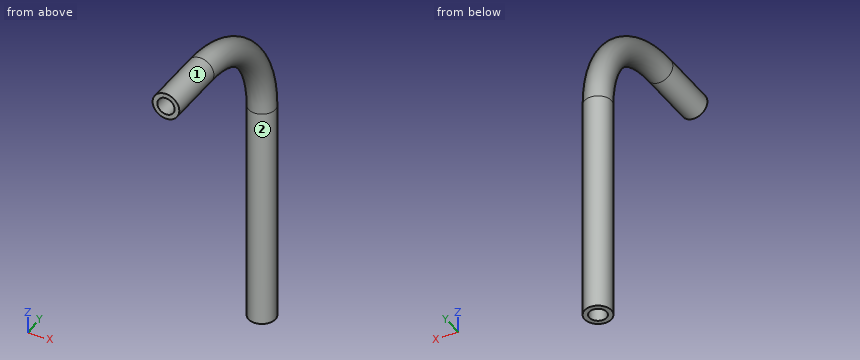
from build123d import *

# Parameters (mm, degrees)
F0_R   = 2
F0_R_2 = 1.3


with BuildPart() as f2:
    # F2: sweep along a path in F1
    with BuildLine(Plane.YZ) as f2_path:
        Line((0, 0), (0, 34))
        ThreePointArc((0, 34), (-4.686291501, 45.313708499), (-16, 50))
        Line((-16, 50), (-25, 50))
    # F0 (on Top) → F2 (sweep)
    with BuildSketch(Plane.XY):
        Circle(F0_R)
        Circle(F0_R_2, mode=Mode.SUBTRACT)
    sweep(path=f2_path.line)


solid = f2.part
Verification items for the finished model (mm, model axes). Face numbers are marked on the shaded views. A direction names the side the tool comes from. Give positions to 0.01 mm unless a question says otherwise; leave off trailing zeros. Write each loop counter-clockwise with the first axis right and the second up, starting at its lowest first coordinate (ties: lowest second). Pieces come first, ordered by that corner, then holes. Notation, with made-up numbers: M -24.75,73.5 L -20.75,73.5 A20 ccw -20.75,90.5 Z; hole C -33.75,-8.75 d9. An arc over 180 degrees is marked long. Write item = value, one per line.
(1) Go/stop test with flat-tipped pins: pin 1 Ø2 at (x, z) = (0, 50) entering from +Y; pin 2 Ø1 at (x, z) = (0.5, 8.5) entering from -Y. Record where each tip stops, or that it passes through.
Found:
pin_1 = -6.05
pin_2 = -2
(2) Material ranges on line 1 (Y direction, x = 0, z = 16); line 2 (Z direction, x = 0, y = -19.25), recorded low to high.
Found:
line_1 = -2 to -1.3, 1.3 to 2
line_2 = 48 to 48.7, 51.3 to 52
(3) Access from +Z, -Z, +X, -X, +Y, -Y to the whole of each face (thin tool, end or side, straight path). Record for the marked faces 1 and 2.
Found:
face_1 = -Y
face_2 = -Z
(4) Sectioned sample at C-C (y = -23). Record the cut outline in (x, z), then the cut area to 3 significant figures.
Found:
outline = C 0,50 d4; hole C 0,50 d2.6
area = 7.26 mm2
(5) Sectioned sample at A-A (x = 0). Record the cut outline in (y, z).
Found:
outline = M -25,48 L -16,48 A14 cw -2,34 L -2,0 L -1.3,0 L -1.3,34 A14.7 ccw -16,48.7 L -25,48.7 Z; M -25,51.3 L -16,51.3 A17.3 cw 1.3,34 L 1.3,0 L 2,0 L 2,34 A18 ccw -16,52 L -25,52 Z
(6) Sectioned sample at B-B (z = 13). Record the cut outline in (x, y).
Found:
outline = C 0,0 d4; hole C 0,0 d2.6
